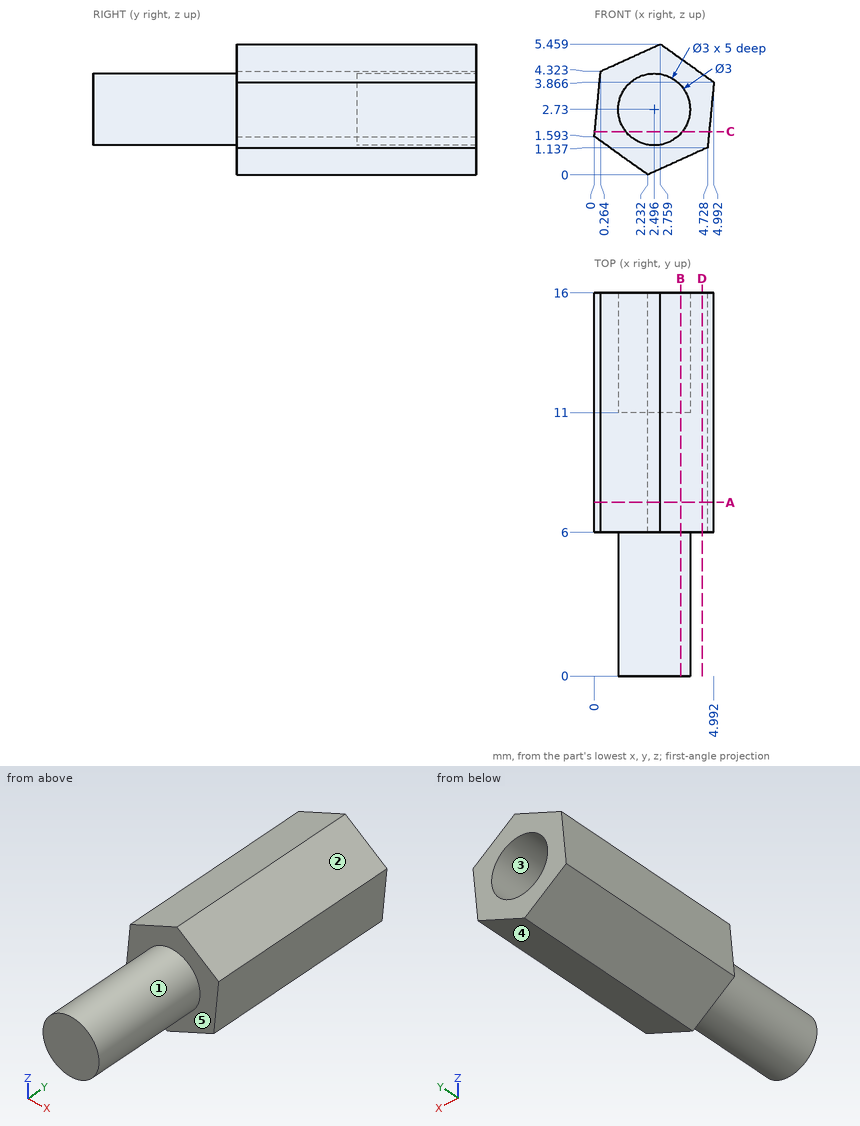
Here's the drawing with two shaded views (mm, measured from the low corner). I have some questions. A direction names the side the tool comes from. Round coordinates to 2 decimals unless told otherwise and drop trailing zeros. Order: outer loops, then holes, each group sorted by start corner. A loop starts at its lowest first (then second) coordinate and runs counter-clockwise, first axis right, second up. Notation, with made-up numbers: (-15.75, 63.25) -> (37.25, 63.25) arc R14 cw to (37.25, 90.25) -> close; hole circle Ø11 at (46, 69). An arc over 180 degrees is marked (long way). Write each question's results on one line, items separated by ' | '. Start each with the question number.
Item 1: Which directions (+Z, -Z, +X, -X, +Y, -Y) give clear straight access to the entire face, cutting with the end or side of a thin tool? Please do the marked faces 1 and 2.
Item 2: If we section it at C-C, the plane z = 1.8: Write out the boundary of the cut face in (x, y).
Item 3: If we section it at D-D, the plane x = 4.5: Write out the boundary of the cut face in (y, z).
Item 4: Will this pin go through, and if not, where does the flat tip stop? pin 1 (1.5 mm diameter, centred on x = 2.5, y = 13.5, fed in from -Z).
Item 5: If we section it at A-A, the plane y = 7.25: Write out the boundary of the cut face in (x, z).
Item 6: If we section it at B-B, the plane x = 3.6: Write out the boundary of the cut face in (y, z) (1 decimal), then the cut area to 3 significant figures.
Item 7: Please list where these lines run through material, in increasing order: L1, parallel to Y at x = 3.15, z = 3.65; L2, parallel to Y at x = 4.55, z = 3.2; L3, parallel to X at y = 2, z = 2.65.
Item 8: Thinking about a two-plate mould opening in Z: for the marked faces 3, 4 and 5, which applies, +Z half, -Z half, draft (parallel to the pull), parting line (faces both ways), or undercut?
Results:
1) face 1: -Y | face 2: +Z, +X, +Y, -Y
2) outline: (0.02, 6) -> (1.32, 6) -> (1.32, 0) -> (3.67, 0) -> (3.67, 6) -> (4.79, 6) -> (4.79, 16) -> (3.67, 16) -> (3.67, 11) -> (1.32, 11) -> (1.32, 16) -> (0.02, 16) -> close
3) outline: (6, 1.03) -> (16, 1.03) -> (16, 4.22) -> (6, 4.22) -> close
4) pin 1: stops at z = 0
5) outline: (0, 1.59) -> (2.23, 0) -> (4.73, 1.14) -> (4.99, 3.87) -> (2.76, 5.46) -> (0.26, 4.32) -> close
6) outline: (0, 1.7) -> (6, 1.7) -> (6, 0.6) -> (16, 0.6) -> (16, 1.7) -> (11, 1.7) -> (11, 3.7) -> (16, 3.7) -> (16, 4.9) -> (6, 4.9) -> (6, 3.7) -> (0, 3.7) -> close | area: 44.4 mm2
7) L1: y = 0 to 11 | L2: y = 6 to 16 | L3: x = 1 to 3.99
8) face 3: undercut | face 4: -Z half | face 5: draft
